```python
from build123d import *

# Parameters (mm, degrees)
BOSS_EXTRUDE1_DEPTH = 1.524
FILLET1_R           = 0.762
FILLET2_R           = 0.762


with BuildPart() as part:
    # Sketch1 → Boss-Extrude1 (new body)
    with BuildSketch(Plane.XY):
        with BuildLine():
            Line((6.433464338, 1.524), (4.909464338, 1.524))
            Line((4.909464338, 1.524), (4.909464338, 0))
            Line((4.909464338, 0), (3.929779176, 0))
            Line((3.929779176, 0), (4.909464338, -2.240840662))
            ThreePointArc((4.909464338, -2.240840662), (6.492968468, -2.870194257), (8.117099911, -3.385721496))
            Line((8.117099911, -3.385721496), (8.449939435, -4.268236242))
            Line((8.449939435, -4.268236242), (8.449939435, -3.47594469))
            ThreePointArc((8.449939435, -3.47594469), (11.023079362, -4.00513675), (13.638615108, -4.250220566))
            Line((13.638615108, -4.250220566), (13.928033002, -5.200165059))
            Line((13.928033002, -5.200165059), (14.121765671, -4.264076161))
            ThreePointArc((14.121765671, -4.264076161), (16.676471214, -4.175606926), (19.207315416, -3.816197909))
            Line((19.207315416, -3.816197909), (19.602084403, -4.268236242))
            Line((19.602084403, -4.268236242), (19.602084403, -3.735071341))
            ThreePointArc((19.602084403, -3.735071341), (21.879297331, -3.128958074), (24.086174716, -2.302662594))
            Line((24.086174716, -2.302662594), (24.468474935, -2.834558551))
            Line((24.468474935, -2.834558551), (24.468474935, -2.133758289))
            ThreePointArc((24.468474935, -2.133758289), (26.244740547, -1.240138243), (27.941024881, -0.202691489))
            Line((27.941024881, -0.202691489), (28.929332922, -0.502746421))
            Line((28.929332922, -0.502746421), (28.474650124, 0.165358914))
            ThreePointArc((28.474650124, 0.165358914), (31.807513974, 3.022993189), (34.564707679, 6.439414997))
            ThreePointArc((34.564707679, 6.439414997), (21.508001683, -1.0948152), (6.433464338, -1.117618174))
            Line((6.433464338, -1.117618174), (7.091019013, 0))
            Line((7.091019013, 0), (6.433464338, 0))
            Line((6.433464338, 0), (6.433464338, 1.524))
        make_face()
    extrude(amount=BOSS_EXTRUDE1_DEPTH)

    # Fillet1
    fillet1_edges = [part.edges().sort_by_distance(p)[0] for p in [
        (6.433464338, -1.117618174, 0.762),
    ]]
    fillet(fillet1_edges, radius=FILLET1_R)

    # Fillet2
    fillet2_edges = [part.edges().sort_by_distance(p)[0] for p in [
        (4.909464338, -2.240840662, 0.762),
    ]]
    fillet(fillet2_edges, radius=FILLET2_R)


solid = part.part
```
Check sheet for the modelled part. Datum: model origin and axes. Units: mm. A direction names the side the tool comes from. Round coordinates to 2 decimals unless told otherwise and drop trailing zeros. Write each loop counter-clockwise with the first axis right and the second up, starting at its lowest first coordinate (ties: lowest second). Pieces come first, ordered by that corner, then holes. Notation, with made-up numbers: (-19.5, -8.5) -> (-7.5, -8.5) arc R32 ccw to (-7.5, 24.5) -> close; hole circle Ø4 at (51.5, 2.25). An arc over 180 degrees is marked (long way). One line per question, with ' | ' between items. Start each with the question number.
1. Set-up check for faces 4 (the face through (6.616, -2.914, 0.751)), 5 (the face through (6.9, -0.9, 0.8)), 6 (the face through (6, 1.524, 1)), 7 (the face through (11, -4, 1)), 8 (the face through (6.433, 1, 1)): record each of +Z, -Z, +X, -X, +Y, -Y from which the full face is reachable in a straight line by a thin tool's end or side.
2. Depth check by flat-ended pin: pin 1 (3 mm diameter, centred on x = 20.5, y = 0.5, fed in from -Z); pin 2 (0.8 mm diameter, centred on y = 1, z = 0.5, fed in from -X); pin 3 (0.5 mm diameter, centred on y = 1, z = 0.5, fed in from +X). Enter the tip coordinate at first touch or a pass-through.
3. Sectioned sample at C-C, the plane y = 5.5. Record the cut outline in (x, z), then the cut area to 3 significant figures.
4. Release check for a two-part mould opening along X. For faces 1 (the face through (28.43, -0.35, 0.75)), 2 (the face through (4.909, 1, 1)), 3 (the face through (16.9, -2.4, 0)) record: +X half, -X half, draft (parallel to the pull), parting line (faces both ways), or undercut.
5. Sectioned sample at A-A, the plane z = 0.25. Record the cut outline in (x, y).
6. Scan lines: line 1 along X through (y, z) = (0.5, 1.3); line 2 along X through (y, z) = (0.75, 0.3); line 3 along Y through (x, z) = (9.5, 0.55). Record each from-to range of solid material in increasing order. Write a range as from..to.
7. Sectioned sample at B-B, the plane x = 32.5. Record the cut outline in (y, z).
Taken from the geometry:
1) face 4: +Z, -Z, -X, -Y | face 5: +Z, -Z | face 6: +Z, -Z, -X, +Y | face 7: +Z, -Z, -Y | face 8: +Z, -Z, +Y
2) pin 1: passes through | pin 2: stops at x = 4.91 | pin 3: stops at x = 29.89
3) outline: (33.58, 0) -> (33.91, 0) -> (33.91, 1.52) -> (33.58, 1.52) -> close | area: 0.500 mm^2
4) face 1: undercut | face 2: -X half | face 3: draft
5) outline: (3.93, 0) -> (4.79, -1.97) arc R0.76 ccw to (5.19, -2.36) arc R24.02 ccw to (8.12, -3.39) -> (8.45, -4.27) -> (8.45, -3.48) arc R24.02 ccw to (13.64, -4.25) -> (13.93, -5.2) -> (14.12, -4.26) arc R24.02 ccw to (19.21, -3.82) -> (19.6, -4.27) -> (19.6, -3.74) arc R24.02 ccw to (24.09, -2.3) -> (24.47, -2.83) -> (24.47, -2.13) arc R24.02 ccw to (27.94, -0.2) -> (28.93, -0.5) -> (28.47, 0.17) arc R24.02 ccw to (34.56, 6.44) arc R29.22 cw to (7.44, -1.37) arc R0.76 cw to (6.95, -0.24) -> (7.09, 0) -> (6.43, 0) -> (6.43, 1.52) -> (4.91, 1.52) -> (4.91, 0) -> close
6) line 1: x = 4.91..6.43, 25.97..28.93 | line 2: x = 4.91..6.43, 26.5..29.26 | line 3: y = -3.73..-1.76
7) outline: (3.77, 0) -> (4.57, 0) -> (4.57, 1.52) -> (3.77, 1.52) -> close
